```python
from build123d import *

# Parameters (mm, degrees)
SKETCH_1_W          = 40
SKETCH_1_H          = 40
EXTRUDE_1_DEPTH     = 3
SKETCH_2_R          = 1.6
CUT_EXTRUDE_1_DEPTH = 29.442925307


with BuildPart() as part:
    # 草图1 → 凸台-拉伸1 (new body)
    with BuildSketch(Plane.XY):
        Rectangle(SKETCH_1_W, SKETCH_1_H)
    extrude(amount=EXTRUDE_1_DEPTH)

    # 草图2 → 切除-拉伸1 (cut, through all)
    with BuildSketch(Plane.XY.offset(3)):
        with Locations((-7.5, 5)):
            Circle(SKETCH_2_R)
        with Locations((7.5, 5)):
            Circle(SKETCH_2_R)
        with Locations((7.5, -5)):
            Circle(SKETCH_2_R)
        with Locations((-7.5, -5)):
            Circle(SKETCH_2_R)
        with Locations((-17, -15)):
            Circle(SKETCH_2_R)
        with Locations((-17, 5)):
            Circle(SKETCH_2_R)
        with Locations(Location((17, 5, 0), (0, 0, 180))):
            Circle(SKETCH_2_R)
        with Locations(Location((17, -15, 0), (0, 0, 180))):
            Circle(SKETCH_2_R)
    extrude(amount=-CUT_EXTRUDE_1_DEPTH, mode=Mode.SUBTRACT)


solid = part.part
```
Build history of the part. All positions in model axes, mm. Give positions to 0.01 mm unless a question says otherwise; leave off trailing zeros. Loops run counter-clockwise (first coordinate to the right, second up) from the corner with the lowest first, then second, coordinate; pieces in that order, holes last.
1) Probe line 1 along Y through (x, z) = (17, 0.95); line 2 along Y through (x, z) = (7.5, 1). List the from-to ranges inside material, lowest first.
Values follow:
line 1: y = -20 to -16.6, -13.4 to 3.4, 6.6 to 20
line 2: y = -20 to -6.6, -3.4 to 3.4, 6.6 to 20
2) Two-plate mould, pull along X, no slides. Class faces 1 (the face through (0, 0, 0)), 2 (the face through (20, 0, 1)), 3 (the face through (5.9, -4.93, 1.52)): released by +X, released by -X, zero draft, split by the parting line, or undercut.
Values follow:
face 1: zero draft
face 2: released by +X
face 3: undercut
3) Band-saw the part on C-C on z = 1.1. State how many separate pieces and enclosed holes the cut face has, then the cut area to 3 significant figures.
Values follow:
separate pieces: 1
enclosed holes: 8
area: 1,540 mm2
4) Band-saw the part on A-A on x = -7.5. List the corners of the cut face in (y, z).
Values follow:
outline: (-20, 0) - (-6.6, 0) - (-6.6, 3) - (-20, 3) - close; (-3.4, 0) - (3.4, 0) - (3.4, 3) - (-3.4, 3) - close; (6.6, 0) - (20, 0) - (20, 3) - (6.6, 3) - close
5) Band-saw the part on B-B on y = -5. List the corners of the cut face in (x, z).
Values follow:
outline: (-20, 0) - (-9.1, 0) - (-9.1, 3) - (-20, 3) - close; (-5.9, 0) - (5.9, 0) - (5.9, 3) - (-5.9, 3) - close; (9.1, 0) - (20, 0) - (20, 3) - (9.1, 3) - close
6) Band-saw the part on D-D on y = 5. List the corners of the cut face in (x, z).
Values follow:
outline: (-20, 0) - (-18.6, 0) - (-18.6, 3) - (-20, 3) - close; (-15.4, 0) - (-9.1, 0) - (-9.1, 3) - (-15.4, 3) - close; (-5.9, 0) - (5.9, 0) - (5.9, 3) - (-5.9, 3) - close; (9.1, 0) - (15.4, 0) - (15.4, 3) - (9.1, 3) - close; (18.6, 0) - (20, 0) - (20, 3) - (18.6, 3) - close
